Check sheet for the modelled part. Datum: model origin and axes. Units: mm. A direction names the side the tool comes from. Round coordinates to 2 decimals unless told otherwise and drop trailing zeros. Order: outer loops, then holes, each group sorted by start corner. A loop starts at its lowest first (then second) coordinate and runs counter-clockwise, first axis right, second up.
(1) Thickness scan on probe 1 along Y at (x, z) = (-4.75, -2.75); probe 2 along Y at (x, z) = (-2.5, 1.5); probe 3 along Z at (x, y) = (2.75, -1.25). Record the ranges inside material, lowest first.
(2) Sectioned sample at D-D, the plane x = 0. Enter the section's corners in (y, z), and give its area (3 significant figures).
(3) Tool access check on faces 5 (the flat face through (0, -3, 0)), 6 (the cylindrical face through (0, -4, -5)), 7 (the flat face through (-4, 0, 0)), 8 (the cylindrical face through (-6.834, -5.986, 1.517)). Record the directions out of +Z, -Z, +X, -X, +Y, -Y that give a thin tool (end or side, any length) a straight path to the whole face; none if there is none.
(4) Sectioned sample at A-A, the plane y = -2. Enter the section's corners in (x, z).
(5) Sectioned sample at C-C, the plane x = -2.5. Enter the section's corners in (y, z), and give its area (3 significant figures).
(6) Mould release check, pull along Y, two halves, no side actions. Record for faces 1 (the flat face through (-2, 2.42, 1.08)), 2 (the cylindrical face through (2.99, -2.44, -0.54)), 3 (the flat face through (0, -7, 0)), 4 (the flat face through (5, -5, 2)): released by +Y, released by -Y, zero draft, split by the parting line, or undercut.
(7) Sectioned sample at B-B, the plane z = 0. Enter the section's corners in (x, y), and give its area (3 significant figures).
(8) Depth check by flat-ended pin: pin 1 (6 mm diameter, centred on y = 0, z = 0, fed in from -X); pin 2 (3 mm diameter, centred on x = -4.5, y = -3, fed in from -Z); pin 3 (3 mm diameter, centred on y = -5, z = -2.5, fed in from +X). Enter the tip coordinate at first touch or a pass-through.
```python
from build123d import *

# Parameters (mm, degrees)
REVOLVE1_ANGLE      = 180
SKETCH2_R           = 5
BOSS_EXTRUDE1_DEPTH = 5
SKETCH3_R           = 7
BOSS_EXTRUDE2_DEPTH = 2
CUT_EXTRUDE1_START  = -3
SKETCH4_W           = 2
SKETCH4_H           = 10
CUT_EXTRUDE1_DEPTH  = 16.124355653
SKETCH6_R           = 2.5
CUT_EXTRUDE2_DEPTH  = 2


with BuildPart() as part:
    # Sketch1 → Revolve1 (revolve)
    with BuildSketch(Plane(origin=(0, 0, 0), x_dir=(1, 0, 0), z_dir=(0, 1, 0))):
        with BuildLine():
            Line((-5, 0), (5, 0))
            ThreePointArc((5, 0), (0, 5), (-5, 0))
        make_face()
    revolve(axis=Axis((-5, 0, 0), (1, 0, 0)), revolution_arc=REVOLVE1_ANGLE)

    # Sketch2 → Boss-Extrude1 (add)
    with BuildSketch(Plane.XZ):
        with Locations(Location((0, 0, 0), (0, 0, 90))):
            Circle(SKETCH2_R)
    extrude(amount=BOSS_EXTRUDE1_DEPTH)

    # Sketch3 → Boss-Extrude2 (add)
    with BuildSketch(Plane.XZ.offset(5)):
        with Locations(Location((0, 0, 0), (0, 0, 270))):
            Circle(SKETCH3_R)
    extrude(amount=BOSS_EXTRUDE2_DEPTH)

    # Sketch4 → Cut-Extrude1 (cut)
    with BuildSketch(Plane(origin=(0, 0, 0), x_dir=(1, 0, 0), z_dir=(0, 1, 0)).offset(CUT_EXTRUDE1_START)):
        with Locations((1, 0)):
            Rectangle(SKETCH4_W, SKETCH4_H)
    cut_extrude1 = extrude(amount=CUT_EXTRUDE1_DEPTH, mode=Mode.SUBTRACT)

    # Sketch6 → Cut-Extrude2 (cut)
    with BuildSketch(Plane.ZY.offset(-2)):
        Circle(SKETCH6_R)
    cut_extrude2 = extrude(amount=-CUT_EXTRUDE2_DEPTH, mode=Mode.SUBTRACT)

    # Mirror1: Cut-Extrude1, Cut-Extrude2 across plane
    add(cut_extrude1.mirror(Plane(origin=(0, 0, 0), x_dir=(0, 0, 1), z_dir=(1, 0, 0))), mode=Mode.SUBTRACT)
    add(cut_extrude2.mirror(Plane(origin=(0, 0, 0), x_dir=(0, 0, 1), z_dir=(1, 0, 0))), mode=Mode.SUBTRACT)


solid = part.part
```
Derived:
1. probe 1: y = -7 to -5
1. probe 2: y = -7 to -2, 2 to 4.06
1. probe 3: z = -4.18 to -2.17, 2.17 to 4.18
2. outline: (-7, -7) - (-5, -7) - (-5, -5) - (-3, -5) - (-3, 5) - (-5, 5) - (-5, 7) - (-7, 7) - close
2. area: 48.0 mm2
3. face 5: +Z, -Z, +Y
3. face 6: +Y
3. face 7: none
3. face 8: +Y, -Y
4. outline: (-4, -1.5) - (-4, 1.5) - (-2, 1.5) - (-2, 4.58) arc R5 ccw to (-2, -4.58) - (-2, -1.5) - close; (2, -4.58) arc R5 ccw to (2, 4.58) - (2, 1.5) - (4, 1.5) - (4, -1.5) - (2, -1.5) - close
5. outline: (-7, -6.54) - (-5, -6.54) - (-5, -4.33) - (0, -4.33) arc R4.33 ccw to (0, 4.33) - (-5, 4.33) - (-5, 6.54) - (-7, 6.54) - close; hole circle Ø5 at (0, 0)
5. area: 79.3 mm2
6. face 1: zero draft
6. face 2: undercut
6. face 3: released by -Y
6. face 4: released by +Y
7. outline: (-7, -7) - (7, -7) - (7, -5) - (5, -5) - (5, 0) arc R5 ccw to (2, 4.58) - (2, 2.5) - (4, 2.5) - (4, -2.5) - (2, -2.5) - (2, -3) - (-2, -3) - (-2, -2.5) - (-4, -2.5) - (-4, 2.5) - (-2, 2.5) - (-2, 4.58) arc R5 ccw to (-5, 0) - (-5, -5) - (-7, -5) - close
7. area: 65.8 mm2
8. pin 1: stops at x = -5
8. pin 2: stops at z = -4
8. pin 3: stops at x = 6.93
